CAD build for the part. Positions are in the model's coordinates, mm. A direction names the side the tool comes from. Round coordinates to 2 decimals unless told otherwise and drop trailing zeros. Write each loop counter-clockwise with the first axis right and the second up, starting at its lowest first coordinate (ties: lowest second). Pieces come first, ordered by that corner, then holes. Notation, with made-up numbers: (65, 31.25) - (70, 31.25) arc R14 cw to (70, 51.25) - close; hole circle Ø5 at (78, 42). An arc over 180 degrees is marked (long way). Use one line per item in the form item = value. Start each with the question number.
Item 1: Band-saw the part on A-A, the plane y = 277. List the corners of the cut face in (x, z).
Item 2: Drill centre lines: L1, parallel to Y at x = 80, z = 2.4; L2, parallel to X at y = -458, z = 3.7; L3, parallel to Y at x = 40, z = 3.4. Where is each one in solid material? Low to high.
Item 3: Tool access for faces 1 (the flat face through (80, 8, 0)), 2 (the flat face through (1, 8, 2)): list every direction of +Z, -Z, +X, -X, +Y, -Y with a clear straight run to the whole face (end or side of a thin tool).
Item 4: Pin check, flat tips, straight feed: pin 1 (1.5 mm diameter, centred on x = 69.5, z = 1, fed in from -Y); pin 2 (2 mm diameter, centred on x = 60, y = 2, fed in from -Z). Stop position of each tip, or through.
Item 5: Band-saw the part on B-B, the plane x = -1. List the corners of the cut face in (y, z).
from build123d import *

# Parameters (mm, degrees)
SKETCH1_W           = 180
SKETCH1_H           = 1200
BOSS_EXTRUDE1_DEPTH = 5
SKETCH2_W           = 140
SKETCH2_H           = 1200
CUT_EXTRUDE1_DEPTH  = 2
SKETCH3_R           = 3.3
CUT_EXTRUDE2_DEPTH  = 6
SKETCH4_R           = 2.5
CUT_EXTRUDE3_DEPTH  = 6


with BuildPart() as part:
    # Sketch1 → Boss-Extrude1 (new body)
    with BuildSketch(Plane.XY):
        Rectangle(SKETCH1_W, SKETCH1_H)
    extrude(amount=BOSS_EXTRUDE1_DEPTH)

    # Sketch2 → Cut-Extrude1 (cut)
    with BuildSketch(Plane(origin=(0, 0, 0), x_dir=(-1, 0, 0), z_dir=(0, 0, -1))):
        Rectangle(SKETCH2_W, SKETCH2_H)
    extrude(amount=-CUT_EXTRUDE1_DEPTH, mode=Mode.SUBTRACT)

    # Sketch3 → Cut-Extrude2 (cut, through all)
    with BuildSketch(Plane.XY.offset(5)):
        with Locations((-40, -521.5)):
            Circle(SKETCH3_R)
        with Locations((-40, -458)):
            Circle(SKETCH3_R)
        with Locations((-40, 585)):
            Circle(SKETCH3_R)
        with Locations((40, 585)):
            Circle(SKETCH3_R)
        with Locations((40, -458)):
            Circle(SKETCH3_R)
        with Locations((40, -521.5)):
            Circle(SKETCH3_R)
    extrude(amount=-CUT_EXTRUDE2_DEPTH, mode=Mode.SUBTRACT)

    # Sketch4 → Cut-Extrude3 (cut, through all)
    with BuildSketch(Plane(origin=(0, 0, 0), x_dir=(-1, 0, 0), z_dir=(0, 0, -1))):
        with Locations((-80, 539.95)):
            Circle(SKETCH4_R)
        with Locations((-80, 529)):
            Circle(SKETCH4_R)
        with Locations((-80, -394.05)):
            Circle(SKETCH4_R)
        with Locations((-80, -405)):
            Circle(SKETCH4_R)
    extrude(amount=-CUT_EXTRUDE3_DEPTH, mode=Mode.SUBTRACT)


solid = part.part
Determined:
q1.outline = (-90, 0) - (-70, 0) - (-70, 2) - (70, 2) - (70, 0) - (90, 0) - (90, 5) - (-90, 5) - close
q2.L1 = -600 to -407.5, -402.5 to -396.55, -391.55 to 526.5, 531.5 to 537.45, 542.45 to 600
q2.L2 = -90 to -43.3, -36.7 to 36.7, 43.3 to 90
q2.L3 = -600 to -524.8, -518.2 to -461.3, -454.7 to 581.7, 588.3 to 600
q3.face_1 = -Z, +X, -X, +Y, -Y
q3.face_2 = -Z, +Y, -Y
q4.pin_1 = -600
q4.pin_2 = 2
q5.outline = (-600, 2) - (600, 2) - (600, 5) - (-600, 5) - close
